Answer from the drawing. Dimensions are ordinates in mm from the lowest x, y and z of the part. A direction names the side the tool comes from. Give positions to 0.01 mm unless a question says otherwise; leave off trailing zeros. Use a Markdown table: item, result. Add a question column.
Q1. For the marked faces 1 and 2, determine the directions among +Z, -Z, +X, -X, +Y, -Y from which every point of the face is accessible in a straight line to the end or side of a thin tool.
Q2. This flat-tipped pin is pushed along its axis until it touches: pin 1 Ø1.5 at (x, y) = (2.5, 0.5) entering from +Z. Where does it stop, or does it pass through?
Q3. Consider line 1 (Y direction, x = 1.85, z = 2.75) (1 decimal); line 2 (Z direction, x = 3.6, y = 2.5); line 3 (Z direction, x = 2.5, y = 4) (1 decimal). Determine where each line is inside the solid, lowest interval first.
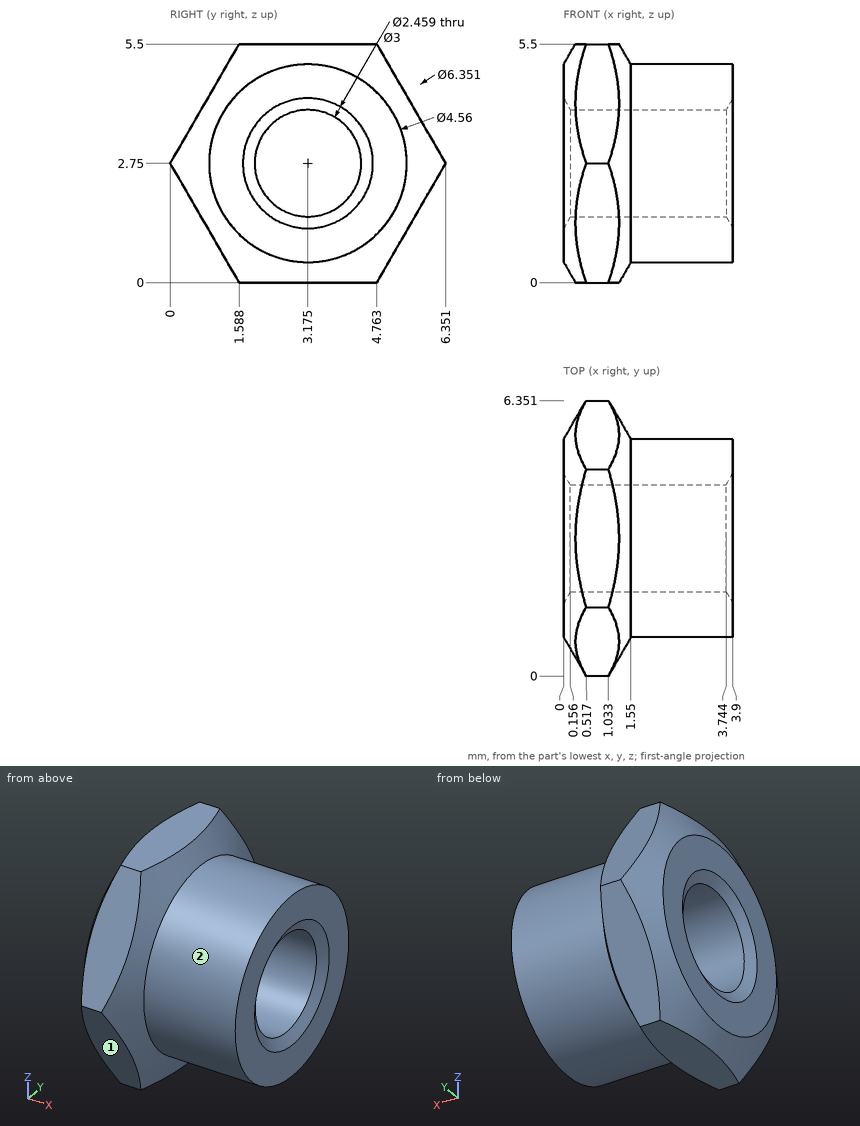
Result set:
| question | item | result |
|---|---|---|
| 1 | face 1 | -Z, +X, -X, -Y |
| 1 | face 2 | +X |
| 2 | pin 1 | stops at z = 3.97 |
| 3 | line 1 | y = 0.9 to 1.9, 4.4 to 5.5 |
| 3 | line 2 | z = 0.57 to 1.72, 3.78 to 4.93 |
| 3 | line 3 | z = 0.6 to 1.8, 3.7 to 4.9 |
